Geometry: see drawing. Coordinates: mm, zero at the bounding-box minimum. Round coordinates to 2 decimals unless told otherwise and drop trailing zeros. Loops run counter-clockwise (first coordinate to the right, second up) from the corner with the lowest first, then second, coordinate; pieces in that order, holes last. Notation, with made-up numbers: (-11, 44) - (11, 44) arc R27 ccw to (11, 80) - close; hole circle Ø6 at (2.5, 1). An arc over 180 degrees is marked (long way). Answer in a Markdown table with one row per item. Add a question column.
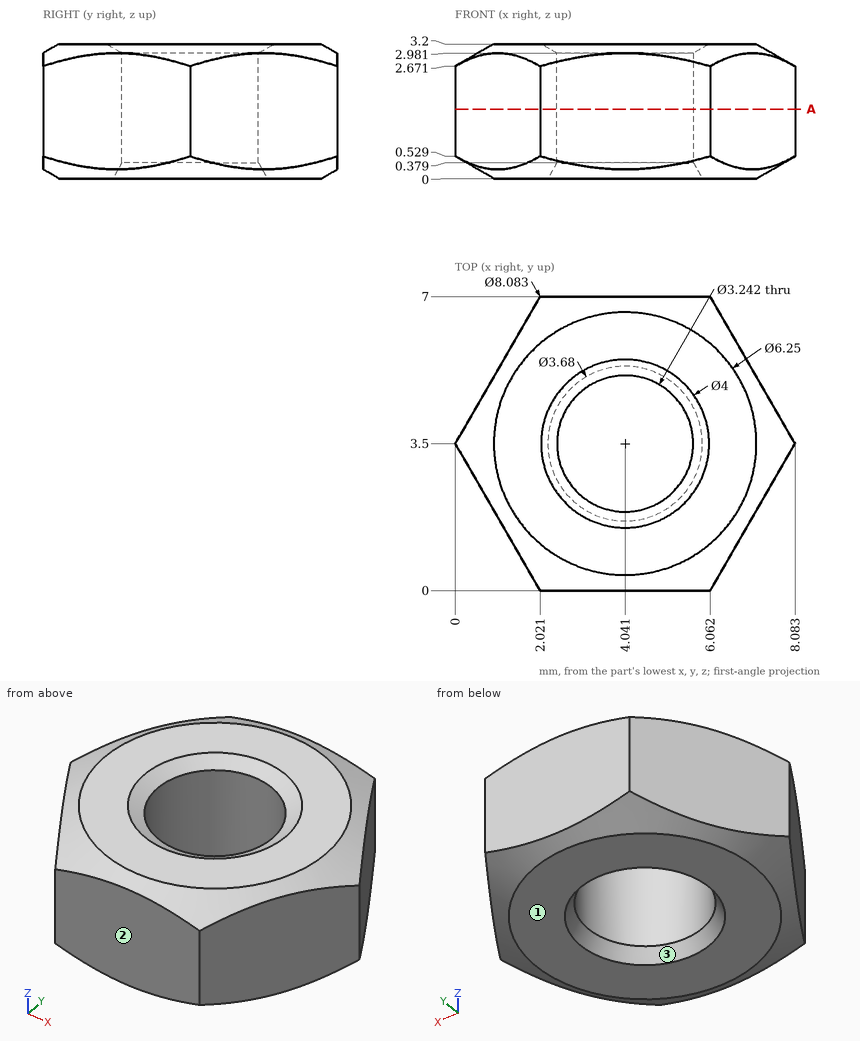
1) Pull-direction query (Y, two-part tool) for the marked faces 1, 2 and 3; classes: pulls with the +Y half, pulls with the -Y half, needs draft (parallel to the pull), parting line crosses it, or undercut.
2) Section A-A, the plane z = 1.65. Return the cut outline in (x, y).
3) Contact query for a flat-ended pin moving along its axis: pin 1 Ø1.5 at (y, z) = (0.5, 2.5) entering from -X. Output: stop coordinate, or through.
4) Material intervals for line 1 along Y through (x, z) = (3.5, 1.9); line 2 along X through (y, z) = (4.75, 1.5) (1 decimal); line 3 along Y through (x, z) = (5, 0.55) (1 decimal), sorted ascending. Write a range as from..to.
Evaluation:
| question | item | result |
|---|---|---|
| 1 | face 1 | needs draft |
| 1 | face 2 | pulls with the -Y half |
| 1 | face 3 | undercut |
| 2 | outline | (0, 3.5) - (2.02, 0) - (6.06, 0) - (8.08, 3.5) - (6.06, 7) - (2.02, 7) - close; hole circle Ø3.24 at (4.04, 3.5) |
| 3 | pin 1 | stops at x = 1.3 |
| 4 | line 1 | y = 0..1.97, 5.03..7 |
| 4 | line 2 | x = 0.7..3, 5.1..7.4 |
| 4 | line 3 | y = 0..2.2, 4.8..7 |
